The figure shows three views and two pictorial views of one solid part (mm, origin at its lowest corner). Answer the questions. Give positions to 0.01 mm unless a question says otherwise; leave off trailing zeros. Order: outer loops, then holes, each group sorted by start corner. A loop starts at its lowest first (then second) coordinate and runs counter-clockwise, first axis right, second up. Notation, with made-up numbers: (-33.5, 47.5) -> (11.5, 47.5) arc R16 cw to (11.5, 75.5) -> close; hole circle Ø8 at (4.25, 87). An arc over 180 degrees is marked (long way). Use one line per item in the form item = value.
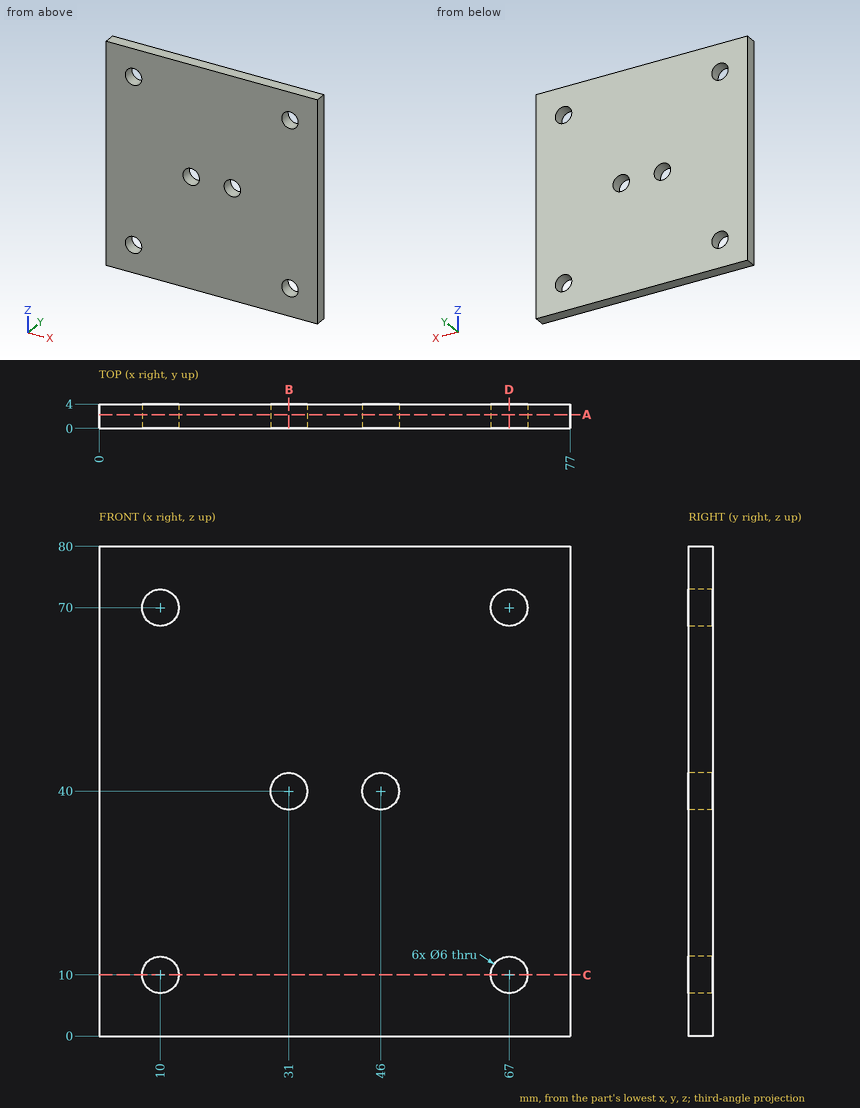
Item 1: Given pin 1 Ø7 at (x, z) = (67, 10) entering from +Y; pin 2 Ø3.5 at (x, z) = (31, 40) entering from -Y, each flat-ended and moving along its own axis, determine where each tip first touches the part or whether it passes through.
Checks:
pin_1 = 4
pin_2 = through
Item 2: The part is cut by section A-A on y = 2.25. Give the vertices of the cut face in (x, z), and give its area (3 significant figures).
Checks:
outline = (0, 0) -> (77, 0) -> (77, 80) -> (0, 80) -> close; hole circle Ø6 at (10, 10); hole circle Ø6 at (10, 70); hole circle Ø6 at (31, 40); hole circle Ø6 at (46, 40); hole circle Ø6 at (67, 10); hole circle Ø6 at (67, 70)
area = 5,990 mm²
Item 3: The part is cut by section C-C on z = 10. Give the vertices of the cut face in (x, y).
Checks:
outline = (0, 0) -> (7, 0) -> (7, 4) -> (0, 4) -> close; (13, 0) -> (64, 0) -> (64, 4) -> (13, 4) -> close; (70, 0) -> (77, 0) -> (77, 4) -> (70, 4) -> close
Item 4: Straight lines are drawn through the part: L1, parallel to X at y = 2.3, z = 10; L2, parallel to X at y = 2.35, z = 40; L3, parallel to Z at x = 69.5, y = 3.3. For each, find the intervals that lie inside material, in ascending order. Write a range as from..to.
Checks:
L1 = 0..7, 13..64, 70..77
L2 = 0..28, 34..43, 49..77
L3 = 0..8.34, 11.66..68.34, 71.66..80
Item 5: The part is cut by section D-D on x = 67. Give the vertices of the cut face in (y, z).
Checks:
outline = (0, 0) -> (4, 0) -> (4, 7) -> (0, 7) -> close; (0, 13) -> (4, 13) -> (4, 67) -> (0, 67) -> close; (0, 73) -> (4, 73) -> (4, 80) -> (0, 80) -> close
Item 6: The part is cut by section B-B on x = 31. Give the vertices of the cut face in (y, z).
Checks:
outline = (0, 0) -> (4, 0) -> (4, 37) -> (0, 37) -> close; (0, 43) -> (4, 43) -> (4, 80) -> (0, 80) -> close
